Autodesk Inventor part; units mm, degrees
ref_plane "YZ Plane" through (0, 0, 0) normal (1, 0, 0) x (0, 1, 0)
ref_plane "XZ Plane" through (0, 0, 0) normal (0, 1, 0) x (-1, 0, 0)
ref_plane "XY Plane" through (0, 0, 0) normal (0, 0, 1) x (1, 0, 0)
sketch "Sketch1" plane through (0, 0, 0) normal (0, 0, 1) x (1, 0, 0)
  circle A0 centre (0, 0) radius 11
  line L0 (-10.583, 3) -> (10.583, 3)
  circle A1 centre (0, 0) radius 15
  line L1 (-14.6969, 3) -> (14.6969, 3)
  dimension "d0" = 22
  dimension "d1" = 3
  dimension "d2" = 4
extrude "Extrusion1" add sketch "Sketch1" along normal blind 40 contours A0 L1 A1 picked at (-0.4305, 13.5639)
sketch "Sketch2" plane through (10.583, 3, 0) normal (0, -1, 0) x (1, 0, 0)
  line L0 (-10.583, 0) -> (9.417, 0)
  line L1 (-10.583, 0) -> (-10.583, 40)
  line L2 (-21.166, 40) -> (0, 40)
  line L3 (-10.583, 20) -> (9.417, 20)
  line L4 (9.417, 20) -> (9.417, 5)
  circle A0 centre (9.417, 5) radius 1.5
  circle A1 centre (9.417, 5) radius 5
  line L5 (0, 0) -> (4.1139, 0)
  line L6 (9.417, 10) -> (4.1139, 10)
  line L7 (4.1139, 10) -> (4.1139, 0)
  line L8 (4.1139, 0) -> (9.417, 0)
  line L9 (9.417, 0) -> (9.417, 10)
  line L10 (-10.583, 40) -> (9.417, 40)
  circle A2 centre (9.417, 35) radius 1.5
  circle A3 centre (9.417, 35) radius 5
  line L11 (9.417, 30) -> (4.1139, 30)
  line L12 (9.417, 40) -> (9.417, 30)
  line L13 (0, 0) -> (4.1139, 0)
  line L14 (4.1139, 0) -> (4.1139, 40)
  line L15 (0, 40) -> (4.1139, 40)
  line L16 (0, 0) -> (0, 40)
  line L17 (4.1139, 30) -> (0, 30)
  line L18 (4.1139, 10) -> (0, 10)
  line L19 (0, 0) -> (0, 40)
  point P0 (0, 20)
  point P1 (4.1139, 20)
  dimension "d8" = 10
  dimension "d5" = 20
  dimension "d6" = 15
  dimension "d7" = 3
extrude "Extrusion2" add sketch "Sketch2" against normal blind 6 contours L16 L18 L7 L0 | L7 L6 A1 L0 | L9 A0 L4 A1 | A1 L4 A0 L9 | L10 L14 L17 L16 | L10 A3 L11 L14 | L12 A2 A3 | A3 L12 A2
mirror "Mirror1" about plane through (0, 0, 0) normal (1, 0, 0) of "Extrusion2"
properties part number "Shaft_conn_Tensioner"
Read the model definition and answer for the solid it produces. Units are mm, in the model's axes. A direction names the side the tool comes from. Coordinates: 2 decimals unless noted, no trailing zeros. Write each loop counter-clockwise with the first axis right and the second up, starting at its lowest first coordinate (ties: lowest second). Pieces come first, ordered by that corner, then holes. Notation, with made-up numbers: (-1.5, -34.5) - (20.5, -34.5) arc R8 cw to (20.5, -28.5) - close; hole circle Ø10 at (23, 7.25). An arc over 180 degrees is marked (long way). Answer as a JSON object with one key per item and string values. Group by question number.
1. A cutting plane is placed at B-B (y = 5.5). Determine the outline of the cut face in (x, z).
2. Consider L1, parallel to Z at x = 20, y = 7.1; L2, parallel to X at y = 6.8, z = 5; L3, parallel to X at y = 6.35, z = 5. Determine where each line is inside the solid, lowest interval first. Write a range as [from, to].
3. A cutting plane is placed at C-C (z = 31). Determine the outline of the cut face in (x, y).
4. A cutting plane is placed at D-D (x = -7.5). Determine the outline of the cut face in (y, z).
5. Which of the six approach directions +Z, -Z, +X, -X, +Y, -Y give full straight-line access (tool end or side, diameter ignored) to faces 5 (the flat face through (17, 6, 30)), 6 (the flat face through (-17, 9, 35)), 7 (the flat face through (18, 9, 5)), 8 (the flat face through (-17, 6, 10))?
6. Each of these flat-tipped pins is pushed along its axis until it touches: P1, Ø4, axis at x = -4, z = 17, coming from the -Y side; P2, Ø4, axis at x = 20, z = 35, coming from the +Y side; P3, Ø4, axis at x = -13, z = 22, coming from the +Y side. Where does it stop, or does it pass through?
7. A cutting plane is placed at A-A (z = 5). Determine the outline of the cut face in (x, y).
8. The mould has two halves that part along X. Classify faces 1 (the cylindrical face through (-25, 6, 35)), 2 (the cylindrical face through (0, 15, 20)), 3 (the cylindrical face through (18.5, 5.96, 5.07)), 4 (the cylindrical face through (-18.5, 5.96, 4.93)): +X half, -X half, draft (parallel to the pull), parting line (faces both ways), or undercut.
Worked out:
{
 "1": {"outline": "(-20, 0) - (-9.53, 0) - (-9.53, 40) - (-20, 40) arc R5 ccw to (-20, 30) - (-13.96, 30) - (-13.96, 10) - (-20, 10) arc R5 ccw to start; (9.53, 0) - (20, 0) arc R5 ccw to (20, 10) - (13.96, 10) - (13.96, 30) - (20, 30) arc R5 ccw to (20, 40) - (9.53, 40) - close; hole circle Ø3 at (-20, 5); hole circle Ø3 at (-20, 35); hole circle Ø3 at (20, 5); hole circle Ø3 at (20, 35)"},
 "2": {"L1": "z = [0, 3.5], [6.5, 10], [30, 33.5], [36.5, 40]", "L2": "x = [-25, -21.5], [-18.5, -8.65], [8.65, 18.5], [21.5, 25]", "L3": "x = [-25, -21.5], [-18.5, -8.98], [8.98, 18.5], [21.5, 25]"},
 "3": {"outline": "(-23, 3) - (-10.58, 3) arc R11 cw to (10.58, 3) - (23, 3) - (23, 9) - (12, 9) arc R15 ccw to (-12, 9) - (-23, 9) - close"},
 "4": {"outline": "(8.05, 0) - (12.99, 0) - (12.99, 40) - (8.05, 40) - close"},
 "5": {"face 5": "+X, +Y", "face 6": "+Z, -Z, -X, +Y", "face 7": "+Z, -Z, +X, +Y", "face 8": "-X, +Y"},
 "6": {"P1": "stops at y = 9.22", "P2": "stops at y = 9", "P3": "stops at y = 10.2"},
 "7": {"outline": "(-25, 3) - (-21.5, 3) - (-21.5, 9) - (-25, 9) - close; (-18.5, 3) - (-10.58, 3) arc R11 cw to (10.58, 3) - (18.5, 3) - (18.5, 9) - (12, 9) arc R15 ccw to (-12, 9) - (-18.5, 9) - close; (21.5, 3) - (25, 3) - (25, 9) - (21.5, 9) - close"},
 "8": {"face 1": "-X half", "face 2": "parting line", "face 3": "undercut", "face 4": "undercut"}
}
